Job drawing, mm, ordinate dimensions from the low corner. One solid piece. A direction names the side the tool comes from. Give positions to 0.01 mm unless a question says otherwise; leave off trailing zeros. Order: outer loops, then holes, each group sorted by start corner. A loop starts at its lowest first (then second) coordinate and runs counter-clockwise, first axis right, second up. Notation, with made-up numbers: M 82.25,53.5 L 129.25,53.5 A16 ccw 129.25,84.5 Z; hole C 58.5,77.5 d4. An arc over 180 degrees is marked long. Put each result on its own line as item: value. Start each with the question number.
1) Pin check, flat tips, straight feed: pin 1 (1.5 mm diameter, centred on x = 3, y = 1, fed in from -Z); pin 2 (2 mm diameter, centred on x = 1.5, z = 1, fed in from +Y). Stop position of each tip, or through.
2) Cut at A-A (y = 2.25). Write the cut outline in (x, z), and give its area (3 significant figures).
3) Tool access for the marked faces 1 and 2: list every direction of +Z, -Z, +X, -X, +Y, -Y with a clear straight run to the whole face (end or side of a thin tool).
4) Drill centre lines: line 1 (Y direction, x = 6.5, z = 3.25); line 2 (Y direction, x = 2, z = 2.2); line 3 (X direction, y = 2.05, z = 2.8). Where is each one in solid material? Low to high. Write a range as [from, to].
5) Cut at C-C (x = 7.75). Write the cut outline in (y, z), and give its area (3 significant figures).
6) Cut at B-B (z = 2.25). Write the cut outline in (x, y).
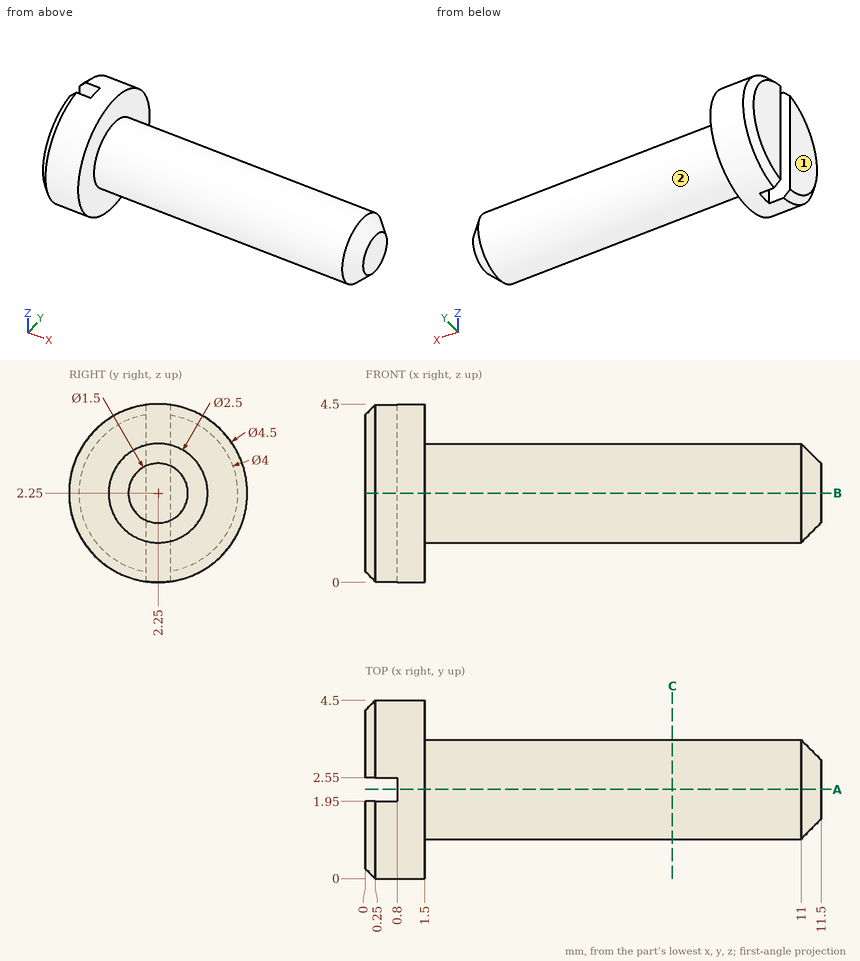
Solution:
1. pin 1: z = 1.1
1. pin 2: y = 4.49
2. outline: M 0.8,0 L 1.5,0 L 1.5,1 L 11,1 L 11.5,1.5 L 11.5,3 L 11,3.5 L 1.5,3.5 L 1.5,4.5 L 0.8,4.5 Z
2. area: 27.9 mm²
3. face 1: +Z, -Z, -X, +Y, -Y
3. face 2: +X
4. line 1: [1.5, 3]
4. line 2: [1, 3.5]
4. line 3: [0.8, 11.5]
5. outline: C 2.25,2.25 d2.5
5. area: 4.91 mm²
6. outline: M 0,0.25 L 0.25,0 L 1.5,0 L 1.5,1 L 11,1 L 11.5,1.5 L 11.5,3 L 11,3.5 L 1.5,3.5 L 1.5,4.5 L 0.25,4.5 L 0,4.25 L 0,2.55 L 0.8,2.55 L 0.8,1.95 L 0,1.95 Z
